Verification items for the finished model (mm, model axes). A direction names the side the tool comes from. Coordinates: 2 decimals unless noted, no trailing zeros. Loops run counter-clockwise (first coordinate to the right, second up) from the corner with the lowest first, then second, coordinate; pieces in that order, holes last. Notation, with made-up numbers: (-19, -6) - (35, -6) arc R16 ccw to (35, -1) - close; hole circle Ø1 at (-1, 44). An arc over 180 degrees is marked (long way). Answer as CSV lines item,"result". Start each with the question number.
1. Cross-section at D-D (y = 2.35). Enter the section's corners in (x, z), plus the area to 3 significant figures.
2. Gauge pin test, flat ends, axial feed: P1, Ø3, axis at x = -18.5, z = -7.5, coming from the -Y side; P2, Ø1.8, axis at x = -3, y = 0.525, coming from the +Z side; P3, Ø0.9, axis at y = 1, z = -8, coming from the +X side. Record the tip position at first contact, or that the pin passes through.
3. Cross-section at B-B (z = -2.5). Enter the section's corners in (x, y) (3 decimals), plus the area to 3 significant figures.
4. Cross-section at A-A (x = -3). Enter the section's corners in (y, z).
5. Cross-section at C-C (y = -0.3). Enter the section's corners in (x, z), plus the area to 3 significant figures.
6. Release check for a two-part mould opening along X. For faces 1 (the flat face through (-8, 1, 0)), 2 (the flat face through (0, 0, -3)), 3 (the flat face through (-13, 1.7, -9.4)), 4 (the cylindrical face through (-1.545, 0.983, -3.451)) record: pulls with the +X half, pulls with the -X half, needs draft (parallel to the pull), parting line crosses it, or undercut.
7. Material ranges on line 1 (Y direction, x = -3, z = -2.75); line 2 (Z direction, x = -4, y = 1.8); line 3 (Y direction, x = -15, z = -3.25), recorded low to high. Write a range as [from, to].
8. Set-up check for faces 5 (the flat face through (-6, 2, -8)), 6 (the flat face through (-18, 2, -9)), 7 (the cylindrical face through (-7.01, -0.71, -3.55)): record each of +Z, -Z, +X, -X, +Y, -Y from which the full face is reachable in a straight line by a thin tool's end or side.
```python
from build123d import *

# Parameters (mm, degrees)
EXTRUDE_1_DEPTH          = 3.5
EXTRUDE_2_DEPTH          = 3.5
EXTRUDE_2_DEPTH_BACK     = 2.45
SKETCH_3_W               = 6
SKETCH_3_H               = 9
CUT_EXTRUDE_1_DEPTH      = 26.244603384
CUT_EXTRUDE_1_DEPTH_BACK = 26.244603384
SKETCH_4_W               = 6
SKETCH_4_H               = 2
SKETCH_5_R               = 1.525
CUT_EXTRUDE_2_DEPTH      = 26.244603384
FILLET_2_R               = 1
FILLET_3_R               = 3


with BuildPart() as part:
    # 草图1 → 凸台-拉伸1 (new body)
    with BuildSketch(Plane(origin=(0, 0, 0), x_dir=(1, 0, 0), z_dir=(0, 1, 0))):
        Polygon((0, 0), (-6, 0), (-15.842640781, 0), (-23, 4.5), (-23, 9), (-13, 9), (-13, 9.8), (-6, 9.8), (-6, 9), (0, 9), align=None)
    extrude(amount=EXTRUDE_1_DEPTH)

    # 草图3 → 凸台-拉伸2 (add, two sides: drawn at the far end of the back side and taken through both)
    with BuildSketch(Plane(origin=(0, 0, 0), x_dir=(1, 0, 0), z_dir=(0, 1, 0)).offset(-EXTRUDE_2_DEPTH_BACK)):
        with Locations((-3, 4.5)):
            Rectangle(SKETCH_3_W, SKETCH_3_H)
    extrude(amount=EXTRUDE_2_DEPTH + EXTRUDE_2_DEPTH_BACK)

    # 草图4 → 切除-拉伸1 (cut, two sides: drawn at the far end of the back side and taken through both)
    with BuildSketch(Plane(origin=(0, 0, 0), x_dir=(1, 0, 0), z_dir=(0, 1, 0)).offset(-CUT_EXTRUDE_1_DEPTH_BACK)):
        with Locations((-3, 8)):
            Rectangle(SKETCH_4_W, SKETCH_4_H)
    extrude(amount=CUT_EXTRUDE_1_DEPTH + CUT_EXTRUDE_1_DEPTH_BACK, mode=Mode.SUBTRACT)

    # 草图5 → 切除-拉伸2 (cut, through all)
    with BuildSketch(Plane.XY):
        with Locations((-3, 0.525)):
            Circle(SKETCH_5_R)
    extrude(amount=-CUT_EXTRUDE_2_DEPTH, mode=Mode.SUBTRACT)

    # 圆角2
    fillet_2_edges = [part.edges().sort_by_distance(p)[0] for p in [
        (-6, 1.75, -9.8),
    ]]
    fillet(fillet_2_edges, radius=FILLET_2_R)

    # 圆角3
    # the kernel refuses this fillet: 3 mm, written as the material it adds along each edge
    with BuildSketch(Plane(origin=(-6, 0, -7), x_dir=(-1, 0, 0), z_dir=(0, 0, 1))) as fillet_3_piece_1:
        with BuildLine():
            CenterArc((2.949152421, 3), FILLET_3_R, 190.563977589, 79.436022411)
            Line((0, 2.45), (0, 0))
            Line((0, 0), (2.949152421, 0))
        make_face()
    extrude(amount=7)


solid = part.part
```
Values follow:
1,outline,"(-23, -9) - (-13, -9) - (-13, -9.8) - (-7, -9.8) arc R1 ccw to (-6, -8.8) - (-6, -7) - (0, -7) - (0, 0) - (-15.84, 0) - (-23, -4.5) - close"
1,area,"184 mm²"
2,P1,"stops at y = 0"
2,P2,"passes through"
2,P3,"stops at x = -6"
3,outline,"(-19.819, 0) - (-8.949, 0) arc R3 cw to (-6, -2.45) - (0, -2.45) - (0, 3.5) - (-19.819, 3.5) - close; hole circle Ø3.05 at (-3, 0.525)"
3,area,"78.6 mm²"
4,outline,"(-2.45, -7) - (-1, -7) - (-1, 0) - (-2.45, 0) - close; (2.05, -7) - (3.5, -7) - (3.5, 0) - (2.05, 0) - close"
5,outline,"(-7.64, -7) - (-4.28, -7) - (-4.28, 0) - (-7.64, 0) - close; (-1.72, -7) - (0, -7) - (0, 0) - (-1.72, 0) - close"
5,area,"35.5 mm²"
6,face 1,"needs draft"
6,face 2,"pulls with the +X half"
6,face 3,"pulls with the -X half"
6,face 4,"undercut"
7,line 1,"y = [-2.45, -1], [2.05, 3.5]"
7,line 2,"z = [-7, 0]"
7,line 3,"y = [0, 3.5]"
8,face 5,"-Z, +X, +Y, -Y"
8,face 6,"-Z, -X, +Y, -Y"
8,face 7,"+Z, -Z, -X, -Y"
